The listing builds one solid part. Answer for the finished solid, in the listing's coordinates (mm). Round coordinates to 2 decimals unless told otherwise and drop trailing zeros. Loops run counter-clockwise (first coordinate to the right, second up) from the corner with the lowest first, then second, coordinate; pieces in that order, holes last. Notation, with made-up numbers: (-2.75, 36.25) - (15.25, 36.25) arc R33 ccw to (15.25, 64.25) - close; hole circle Ø4 at (71.25, -37.5). An arc over 180 degrees is marked (long way). One line per item, written item: value.
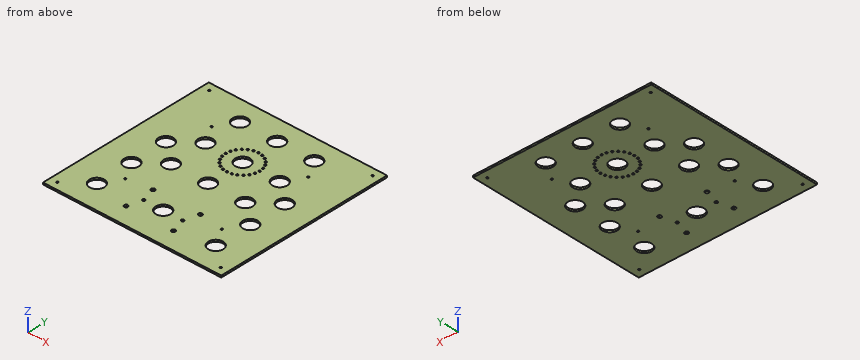
```python
from build123d import *

# Parameters (mm, degrees)
F0_W     = 304.8
F0_H     = 304.8
F0_R     = 1.5875
F0_R_2   = 12.7
F0_R_3   = 3.175
F0_R_4   = 2.38125
F0_R_5   = 1.656096
F1_DEPTH = 3.175


with BuildPart() as f1:
    # F0 (on Top) → F1 (new body)
    with BuildSketch(Plane.XY):
        Rectangle(F0_W, F0_H)
        with Locations((-139.7, -139.7)):
            Circle(F0_R, mode=Mode.SUBTRACT)
        with Locations((-101.6, -107.95)):
            Circle(F0_R_2, mode=Mode.SUBTRACT)
        with Locations((-40.48125, -120.015)):
            Circle(F0_R_3, mode=Mode.SUBTRACT)
        with Locations((-33.3375, -95.25)):
            Circle(F0_R_4, mode=Mode.SUBTRACT)
        with Locations((-82.55, -76.2)):
            Circle(F0_R, mode=Mode.SUBTRACT)
        with Locations((-101.6, -44.45)):
            Circle(F0_R_2, mode=Mode.SUBTRACT)
        with Locations((-40.48125, -70.485)):
            Circle(F0_R_3, mode=Mode.SUBTRACT)
        with Locations((-63.5, -12.7)):
            Circle(F0_R_2, mode=Mode.SUBTRACT)
        with Locations((40.48125, -120.015)):
            Circle(F0_R_3, mode=Mode.SUBTRACT)
        with Locations((0, -95.25)):
            Circle(F0_R_2, mode=Mode.SUBTRACT)
        with Locations((33.3375, -95.25)):
            Circle(F0_R_4, mode=Mode.SUBTRACT)
        with Locations((139.7, -139.7)):
            Circle(F0_R, mode=Mode.SUBTRACT)
        with Locations((101.6, -107.95)):
            Circle(F0_R_2, mode=Mode.SUBTRACT)
        with Locations((40.48125, -70.485)):
            Circle(F0_R_3, mode=Mode.SUBTRACT)
        with Locations((0, -12.7)):
            Circle(F0_R_2, mode=Mode.SUBTRACT)
        with Locations((63.5, -12.7)):
            Circle(F0_R_2, mode=Mode.SUBTRACT)
        with Locations((82.55, -76.2)):
            Circle(F0_R, mode=Mode.SUBTRACT)
        with Locations((101.6, -44.45)):
            Circle(F0_R_2, mode=Mode.SUBTRACT)
        with Locations((-101.6, 19.05)):
            Circle(F0_R_2, mode=Mode.SUBTRACT)
        with Locations((-20.506097, 30.293903)):
            Circle(F0_R_5, mode=Mode.SUBTRACT)
        with Locations((-25.114737, 36.3)):
            Circle(F0_R_5, mode=Mode.SUBTRACT)
        with Locations((-14.5, 25.685263)):
            Circle(F0_R_5, mode=Mode.SUBTRACT)
        with Locations((-7.505752, 22.788151)):
            Circle(F0_R_5, mode=Mode.SUBTRACT)
        with Locations((-63.5, 50.8)):
            Circle(F0_R_2, mode=Mode.SUBTRACT)
        with Locations((-28.011849, 43.294248)):
            Circle(F0_R_5, mode=Mode.SUBTRACT)
        with Locations((-29, 50.8)):
            Circle(F0_R_5, mode=Mode.SUBTRACT)
        with Locations((-28.011849, 58.305752)):
            Circle(F0_R_5, mode=Mode.SUBTRACT)
        with Locations((-25.114737, 65.3)):
            Circle(F0_R_5, mode=Mode.SUBTRACT)
        with Locations((-20.506097, 71.306097)):
            Circle(F0_R_5, mode=Mode.SUBTRACT)
        with Locations((-14.5, 75.914737)):
            Circle(F0_R_5, mode=Mode.SUBTRACT)
        with Locations((-82.55, 82.55)):
            Circle(F0_R, mode=Mode.SUBTRACT)
        with Locations((-139.7, 139.7)):
            Circle(F0_R, mode=Mode.SUBTRACT)
        with Locations((-7.505752, 78.811849)):
            Circle(F0_R_5, mode=Mode.SUBTRACT)
        with Locations((-63.5, 114.3)):
            Circle(F0_R_2, mode=Mode.SUBTRACT)
        with Locations((0, 21.8)):
            Circle(F0_R_5, mode=Mode.SUBTRACT)
        with Locations((7.505752, 22.788151)):
            Circle(F0_R_5, mode=Mode.SUBTRACT)
        with Locations((14.5, 25.685263)):
            Circle(F0_R_5, mode=Mode.SUBTRACT)
        with Locations((20.506097, 30.293903)):
            Circle(F0_R_5, mode=Mode.SUBTRACT)
        with Locations((25.114737, 36.3)):
            Circle(F0_R_5, mode=Mode.SUBTRACT)
        with Locations((0, 50.8)):
            Circle(F0_R_2, mode=Mode.SUBTRACT)
        with Locations((28.011849, 43.294248)):
            Circle(F0_R_5, mode=Mode.SUBTRACT)
        with Locations((29, 50.8)):
            Circle(F0_R_5, mode=Mode.SUBTRACT)
        with Locations((14.5, 75.914737)):
            Circle(F0_R_5, mode=Mode.SUBTRACT)
        with Locations((28.011849, 58.305752)):
            Circle(F0_R_5, mode=Mode.SUBTRACT)
        with Locations((25.114737, 65.3)):
            Circle(F0_R_5, mode=Mode.SUBTRACT)
        with Locations((20.506097, 71.306097)):
            Circle(F0_R_5, mode=Mode.SUBTRACT)
        with Locations((63.5, 50.8)):
            Circle(F0_R_2, mode=Mode.SUBTRACT)
        with Locations((101.6, 19.05)):
            Circle(F0_R_2, mode=Mode.SUBTRACT)
        with Locations((0, 79.8)):
            Circle(F0_R_5, mode=Mode.SUBTRACT)
        with Locations((7.505752, 78.811849)):
            Circle(F0_R_5, mode=Mode.SUBTRACT)
        with Locations((0, 114.3)):
            Circle(F0_R_2, mode=Mode.SUBTRACT)
        with Locations((63.5, 114.3)):
            Circle(F0_R_2, mode=Mode.SUBTRACT)
        with Locations((82.55, 82.55)):
            Circle(F0_R, mode=Mode.SUBTRACT)
        with Locations((139.7, 139.7)):
            Circle(F0_R, mode=Mode.SUBTRACT)
    extrude(amount=F1_DEPTH)


solid = f1.part
```
1) A cutting plane is placed at D-D on z = 0.8. Give the number of separate pieces and of enclosed holes in the cut face, and give its area (3 significant figures).
Final values:
separate pieces: 1
enclosed holes: 54
area: 84,400 mm2
2) Consider L1, parallel to X at y = 36.5, z = 2.6; L2, parallel to Y at x = -59, z = 1.1; L3, parallel to Y at x = 10.5, z = 1.1. Determine where each line is inside the solid, lowest interval first.
Final values:
L1: -152.4 to -26.76, -23.47 to 23.47, 26.76 to 152.4
L2: -152.4 to -24.58, -0.82 to 38.92, 62.68 to 102.42, 126.18 to 152.4
L3: -152.4 to -102.39, -88.11 to -19.84, -5.56 to 43.66, 57.94 to 107.16, 121.44 to 152.4
3) A cutting plane is placed at C-C on y = -113. Give the vertices of the cut face in (x, z) (3 decimals), and give its area (3 significant figures).
Final values:
outline: (-152.4, 0) - (-113.253, 0) - (-113.253, 3.175) - (-152.4, 3.175) - close; (-89.947, 0) - (89.947, 0) - (89.947, 3.175) - (-89.947, 3.175) - close; (113.253, 0) - (152.4, 0) - (152.4, 3.175) - (113.253, 3.175) - close
area: 820 mm2
4) A cutting plane is placed at B-B on x = -101.6. Give the vertices of the cut face in (y, z) (3 decimals), and give its area (3 significant figures).
Final values:
outline: (-152.4, 0) - (-120.65, 0) - (-120.65, 3.175) - (-152.4, 3.175) - close; (-95.25, 0) - (-57.15, 0) - (-57.15, 3.175) - (-95.25, 3.175) - close; (-31.75, 0) - (6.35, 0) - (6.35, 3.175) - (-31.75, 3.175) - close; (31.75, 0) - (152.4, 0) - (152.4, 3.175) - (31.75, 3.175) - close
area: 726 mm2
5) This flat-tipped pin is pushed along its axis until it touches: pin 1 Ø23 at (x, y) = (-101.6, -107.95) entering from -Z. Where does it stop, or does it pass through?
Final values:
pin 1: through
6) A cutting plane is placed at A-A on y = -44.45. Give the vertices of the cut face in (x, z) (3 decimals), and give its area (3 significant figures).
Final values:
outline: (-152.4, 0) - (-114.3, 0) - (-114.3, 3.175) - (-152.4, 3.175) - close; (-88.9, 0) - (88.9, 0) - (88.9, 3.175) - (-88.9, 3.175) - close; (114.3, 0) - (152.4, 0) - (152.4, 3.175) - (114.3, 3.175) - close
area: 806 mm2
